from build123d import *

# Parameters (mm, degrees)
F0_R     = 7.5
F1_DEPTH = 2
F3_DEPTH = 2


with BuildPart() as f1:
    # F0 (on Top) → F1 (new body)
    with BuildSketch(Plane.XY):
        Circle(F0_R)
    extrude(amount=F1_DEPTH)

    # F2 (on face) → F3 (join)
    with BuildSketch(Plane.XY.offset(2)):
        with BuildLine():
            ThreePointArc((-1.634316, -5.22253), (-0.792326, -5.735097), (0, -6.321519))
            ThreePointArc((0, -6.321519), (0.792326, -5.735097), (1.634316, -5.22253))
            ThreePointArc((1.634316, -5.22253), (3.895395, -3.034618), (4.726373, 0))
            Line((4.726373, 0), (4.726373, 4.415748))
            ThreePointArc((4.726373, 4.415748), (2.363187, 3.860301), (0, 4.415748))
            ThreePointArc((0, 4.415748), (-2.363187, 3.860301), (-4.726373, 4.415748))
            Line((-4.726373, 4.415748), (-4.726373, 0))
            ThreePointArc((-4.726373, 0), (-3.895395, -3.034618), (-1.634316, -5.22253))
        make_face()
    extrude(amount=F3_DEPTH)


solid = f1.part
Verification items for the finished model (mm, model axes). A direction names the side the tool comes from. Coordinates: 2 decimals unless noted, no trailing zeros. Order: outer loops, then holes, each group sorted by start corner. A loop starts at its lowest first (then second) coordinate and runs counter-clockwise, first axis right, second up. Notation, with made-up numbers: (6, 56) -> (54, 56) arc R25 cw to (54, 92) -> close; hole circle Ø3 at (-21.75, 52). An arc over 180 degrees is marked (long way). Put each result on its own line as item: value. Start each with the question number.
1. Access from +Z, -Z, +X, -X, +Y, -Y to the whole of each face (thin tool, end or side, straight path). Record for faces 1 (the flat face through (4.726, 2, 3)), 2 (the cylindrical face through (-7.493, 0.33, 0.986)), 3 (the flat face through (-4.726, 2, 3)), 4 (the cylindrical face through (0.781, -5.743, 2.986)), 5 (the cylindrical face through (-3.918, -2.996, 2.986)).
2. Material ranges on L1, parallel to Z at x = -5.25, y = 0.5; L2, parallel to Y at x = 3, z = 0.85; L3, parallel to X at y = -2.75, z = 2.85, recorded low to high. Write a range as [from, to].
3. Mould release check, pull along X, two halves, no side actions. Record for faces 6 (the cylindrical face through (-0.8, -5.73, 2.99)), 7 (the cylindrical face through (-2.33, 3.86, 2.99)), 8 (the cylindrical face through (2.4, 3.86, 2.99)), 9 (the cylindrical face through (3.873, -3.073, 2.986)): released by +X, released by -X, zero draft, split by the parting line, or undercut.
4. Go/stop test with flat-tipped pins: pin 1 Ø5 at (x, y) = (3, -2.5) entering from -Z; pin 2 Ø1.5 at (y, z) = (-3.5, 1) entering from +X; pin 3 Ø2 at (y, z) = (3, 2.5) entering from -X; pin 4 Ø2 at (y, z) = (2.5, 3.5) entering from +X. Record where each tip stops, or that it passes through.
5. Cross-section at A-A, the plane z = 3.25. Record the boundary of the cut face in (x, y).
6. Cross-section at B-B, the plane y = 0.75. Record the boundary of the cut face in (x, z), then the cut area to 3 significant figures.
7. Cross-section at C-C, the plane z = 0.4. Record the boundary of the cut face in (x, y).
Computed:
1. face 1: +Z, +X, +Y, -Y
1. face 2: +Z, -Z
1. face 3: +Z, -X, +Y, -Y
1. face 4: +Z, +X, -Y
1. face 5: +Z, -X, -Y
2. L1: [0, 2]
2. L2: [-6.87, 6.87]
2. L3: [-4.05, 4.05]
3. face 6: released by -X
3. face 7: undercut
3. face 8: undercut
3. face 9: released by +X
4. pin 1: z = 0
4. pin 2: x = 6.98
4. pin 3: x = -7.19
4. pin 4: x = 4.73
5. outline: (-4.73, 0) arc R5.96 ccw to (-1.63, -5.22) arc R10.92 cw to (0, -6.32) arc R10.92 cw to (1.63, -5.22) arc R5.96 ccw to (4.73, 0) -> (4.73, 4.42) arc R5.3 cw to (0, 4.42) arc R5.3 cw to (-4.73, 4.42) -> close
6. outline: (-7.46, 0) -> (7.46, 0) -> (7.46, 2) -> (4.73, 2) -> (4.73, 4) -> (-4.73, 4) -> (-4.73, 2) -> (-7.46, 2) -> close
6. area: 48.8 mm2
7. outline: circle Ø15 at (0, 0)
